Could you check a few things on this model? Use its own coordinates, in mm. Face numbers are marked on the shaded views. Coordinates: 2 decimals unless noted, no trailing zeros. Write each loop counter-clockwise with the first axis right and the second up, starting at its lowest first coordinate (ties: lowest second). Pieces come first, ordered by that corner, then holes. Notation, with made-up numbers: (66.25, 15) - (70.25, 15) arc R13 ccw to (70.25, 38) - close; hole circle Ø6 at (80, 42.25). An arc over 180 degrees is marked (long way). Answer as a JSON object with one key per item and string values. Group by question number.
1) If we section it at A-A (x = 0): Write out the boundary of the cut face in (y, z), plus the area to 3 significant figures.
2) We'd pull the mould along Z, two halves only. Please class the marked faces 1, 2 and 3: released by +Z, released by -Z, zero draft, split by the parting line, or undercut.
3) Please list where these lines run through material, in increasing order: line 1 along X through (y, z) = (1, 0); line 2 along Y through (x, z) = (-5, -8.75); line 3 along X through (y, z) = (2.2, -8).
4) If we section it at B-B (x = 8): Write out the boundary of the cut face in (y, z), plus the area to 3 significant figures.
5) If we section it at D-D (z = -8): Write out the boundary of the cut face in (x, y).
6) Will these pins go through, and if not, where does the flat tip stop? pin 1 Ø2 at (y, z) = (6, 1) entering from -X; pin 2 Ø4 at (x, y) = (5, 13) entering from -Z; pin 3 Ø8 at (x, z) = (8, 5.5) entering from -Y; pin 4 Ø1 at (x, z) = (-7.5, 6) entering from +Y.
7) If we section it at C-C (z = -0.5): Write out the boundary of the cut face in (x, y), plus the area to 3 significant figures.
```python
from build123d import *

# Parameters (mm, degrees)
SKETCH1_R           = 11
SKETCH1_R_2         = 1
BOSS_EXTRUDE1_DEPTH = 3
SKETCH2_R           = 4
BOSS_EXTRUDE2_DEPTH = 12.7


with BuildPart() as part:
    # Sketch1 → Boss-Extrude1 (new body)
    with BuildSketch(Plane(origin=(0, 0, 0), x_dir=(1, 0, 0), z_dir=(0, 1, 0))):
        with Locations(Location((0, 0, 0), (0, 0, 270))):
            Circle(SKETCH1_R)
        with Locations(Location((0, 8, 0), (0, 0, 270))):
            Circle(SKETCH1_R_2, mode=Mode.SUBTRACT)
        with Locations(Location((8, 0, 0), (0, 0, 270))):
            Circle(SKETCH1_R_2, mode=Mode.SUBTRACT)
        with Locations(Location((0, -8, 0), (0, 0, 270))):
            Circle(SKETCH1_R_2, mode=Mode.SUBTRACT)
        with Locations(Location((-8, 0, 0), (0, 0, 270))):
            Circle(SKETCH1_R_2, mode=Mode.SUBTRACT)
    extrude(amount=BOSS_EXTRUDE1_DEPTH)

    # Sketch2 → Boss-Extrude2 (add)
    with BuildSketch(Plane(origin=(0, 3, 0), x_dir=(1, 0, 0), z_dir=(0, 1, 0))):
        with Locations(Location((0, 0, 0), (0, 0, 270))):
            Circle(SKETCH2_R)
    extrude(amount=BOSS_EXTRUDE2_DEPTH)


solid = part.part
```
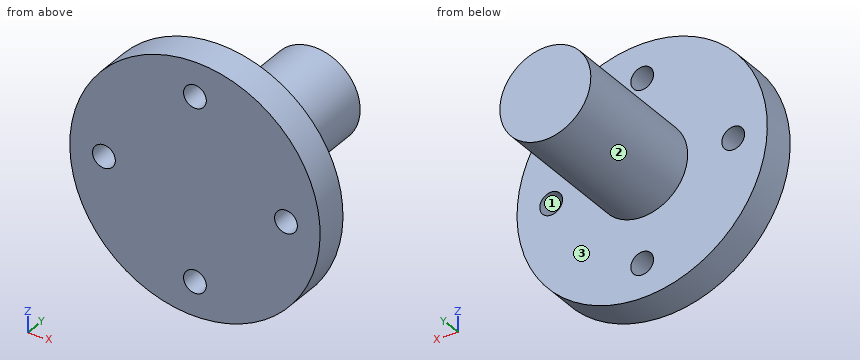
Here are the results:
{
 "1": {"outline": "(0, -11) - (3, -11) - (3, -9) - (0, -9) - close; (0, -7) - (3, -7) - (3, -4) - (15.7, -4) - (15.7, 4) - (3, 4) - (3, 7) - (0, 7) - close; (0, 9) - (3, 9) - (3, 11) - (0, 11) - close", "area": "156 mm²"},
 "2": {"face 1": "undercut", "face 2": "split by the parting line", "face 3": "zero draft"},
 "3": {"line 1": "x = -11 to -9, -7 to 7, 9 to 11", "line 2": "y = 0 to 3", "line 3": "x = -7.55 to -1, 1 to 7.55"},
 "4": {"outline": "(0, -7.55) - (3, -7.55) - (3, -1) - (0, -1) - close; (0, 1) - (3, 1) - (3, 7.55) - (0, 7.55) - close", "area": "39.3 mm²"},
 "5": {"outline": "(-7.55, 0) - (-1, 0) - (-1, 3) - (-7.55, 3) - close; (1, 0) - (7.55, 0) - (7.55, 3) - (1, 3) - close"},
 "6": {"pin 1": "stops at x = -4", "pin 2": "stops at z = -2.65", "pin 3": "stops at y = 0", "pin 4": "stops at y = 3"},
 "7": {"outline": "(-10.99, 0) - (-8.87, 0) - (-8.87, 3) - (-10.99, 3) - close; (-7.13, 0) - (7.13, 0) - (7.13, 3) - (3.97, 3) - (3.97, 15.7) - (-3.97, 15.7) - (-3.97, 3) - (-7.13, 3) - close; (8.87, 0) - (10.99, 0) - (10.99, 3) - (8.87, 3) - close", "area": "156 mm²"}
}
